Work out the finished part from the listing and answer in its coordinate system (mm). A direction names the side the tool comes from. Round coordinates to 2 decimals unless told otherwise and drop trailing zeros. Write each loop counter-clockwise with the first axis right and the second up, starting at its lowest first coordinate (ties: lowest second). Pieces come first, ordered by that corner, then holes.
1. Find section A-A (x = 0). Write down the section's boundary in (y, z).
2. Determine the mould class of faces 1 (the face through (-2, 2, 25.4)), 2 (the face through (70.75, -78.53, 3.49)), 3 (the face through (-114.19, 5.03, 3.49)) for opening direction Y: pulls with the +Y half, pulls with the -Y half, needs draft (parallel to the pull), parting line crosses it, or undercut.
3. Flat-ended cylindrical pins translate along their axes: pin 1 Ø21.5 at (x, y) = (-67.17, 67.17) entering from -Z; pin 2 Ø1.5 at (y, z) = (87, 7.5) entering from +X; pin 3 Ø3 at (x, z) = (-47.5, -15.5) entering from +Y; pin 4 Ø1.5 at (y, z) = (-35, -14.5) entering from -X. Find the tip coordinate at first contact, or state that the pin passes through.
4. Find section D-D (x = 87). Write down the section's boundary in (y, z).
5. Straight lines are drawn through the part: probe 1 along Y at (x, z) = (0, -17); probe 2 along X at (y, z) = (57.5, 5.5); probe 3 along Y at (x, z) = (65, 19.5). For each, find the intervals that lie inside material, in ascending order.
6. A tool of negligible diameter and unlimited length cuts with its end or side. For faces 4 (the face through (-78.53, -70.75, 3.49)), 5 (the face through (52, -52, -16.485)), from which of +Z, -Z, +X, -X, +Y, -Y can it reach the whole face along a straight path? Write none if from no direction.
7. Find section B-B (y = 44.5). Write down the section's boundary in (x, z).
8. Find section C-C (z = 6). Write down the section's boundary in (x, y).
```python
from build123d import *

# Parameters (mm, degrees)
SKETCH1_R           = 114.3
BOSS_EXTRUDE1_DEPTH = 25.4
CUT_EXTRUDE1_START  = -6.35
SKETCH2_R           = 114.3
SKETCH2_R_2         = 68.2498
CUT_EXTRUDE1_DEPTH  = 6.35
SKETCH3_R           = 77.9399
SKETCH3_R_2         = 73.3679
CUT_EXTRUDE2_DEPTH  = 2.5654
CUT_EXTRUDE3_REACH  = 171.439
SKETCH5_R           = 11.90625
CIRPATTERN1_COUNT   = 4


with BuildPart() as part:
    # Sketch1 → Boss-Extrude1 (new, symmetric)
    with BuildSketch(Plane.XY):
        Circle(SKETCH1_R)
    extrude(amount=BOSS_EXTRUDE1_DEPTH, both=True)

    # Sketch2 → Cut-Extrude1 (cut)
    with BuildSketch(Plane(origin=(0, 0, -25.4), x_dir=(-1, 0, 0), z_dir=(0, 0, -1)).offset(CUT_EXTRUDE1_START)):
        Circle(SKETCH2_R)
        Circle(SKETCH2_R_2, mode=Mode.SUBTRACT)
    extrude(amount=CUT_EXTRUDE1_DEPTH, mode=Mode.SUBTRACT)

    # Sketch3 → Cut-Extrude2 (cut)
    with BuildSketch(Plane(origin=(0, 0, -19.05), x_dir=(-1, 0, 0), z_dir=(0, 0, -1))):
        Circle(SKETCH3_R)
        Circle(SKETCH3_R_2, mode=Mode.SUBTRACT)
    extrude(amount=-CUT_EXTRUDE2_DEPTH, mode=Mode.SUBTRACT)

    # Sketch5 → Cut-Extrude3 (cut, up to next)
    with BuildSketch(Plane.XY.offset(25.4), mode=Mode.PRIVATE) as cut_extrude3_sk1:
        with Locations((67.172315786, 67.172315786)):
            Circle(SKETCH5_R)
    cut_extrude3_tool1 = extrude(cut_extrude3_sk1.sketch, amount=-CUT_EXTRUDE3_REACH, mode=Mode.PRIVATE) & part.part
    cut_extrude3 = cut_extrude3_tool1.solids().sort_by_distance((67.172316, 67.172316, 25.4))[0]
    add(cut_extrude3, mode=Mode.SUBTRACT)

    # CirPattern1: Cut-Extrude3 ×4 about axis
    cirpattern1_axis = Axis((0, 0, 0), (0, 0, 1))
    for i in range(1, CIRPATTERN1_COUNT):
        add(cut_extrude3.rotate(cirpattern1_axis, i * 360 / CIRPATTERN1_COUNT), mode=Mode.SUBTRACT)


solid = part.part
```
Worked answers:
1. outline: (-114.3, -19.05) - (-77.94, -19.05) - (-77.94, -16.48) - (-73.37, -16.48) - (-73.37, -19.05) - (-68.25, -19.05) - (-68.25, -25.4) - (68.25, -25.4) - (68.25, -19.05) - (73.37, -19.05) - (73.37, -16.48) - (77.94, -16.48) - (77.94, -19.05) - (114.3, -19.05) - (114.3, 25.4) - (-114.3, 25.4) - close
2. face 1: needs draft
2. face 2: undercut
2. face 3: parting line crosses it
3. pin 1: passes through
3. pin 2: stops at x = 75
3. pin 3: stops at y = 104.64
3. pin 4: stops at x = -109.05
4. outline: (-74.13, -19.05) - (74.13, -19.05) - (74.13, 25.4) - (-74.13, 25.4) - close
5. probe 1: y = -114.3 to -77.94, -73.37 to 73.37, 77.94 to 114.3
5. probe 2: x = -98.78 to -74.12, -60.23 to 60.23, 74.12 to 98.78
5. probe 3: y = -94.02 to -78.88, -55.47 to 55.47, 78.88 to 94.02
6. face 4: +Z, -Z
6. face 5: -Z
7. outline: (-105.28, -19.05) - (-63.99, -19.05) - (-63.99, -16.48) - (-58.33, -16.48) - (-58.33, -19.05) - (-51.75, -19.05) - (-51.75, -25.4) - (51.75, -25.4) - (51.75, -19.05) - (58.33, -19.05) - (58.33, -16.48) - (63.99, -16.48) - (63.99, -19.05) - (105.28, -19.05) - (105.28, 25.4) - (-105.28, 25.4) - close
8. outline: circle Ø228.6 at (0, 0); hole circle Ø23.81 at (-67.17, -67.17); hole circle Ø23.81 at (-67.17, 67.17); hole circle Ø23.81 at (67.17, -67.17); hole circle Ø23.81 at (67.17, 67.17)
